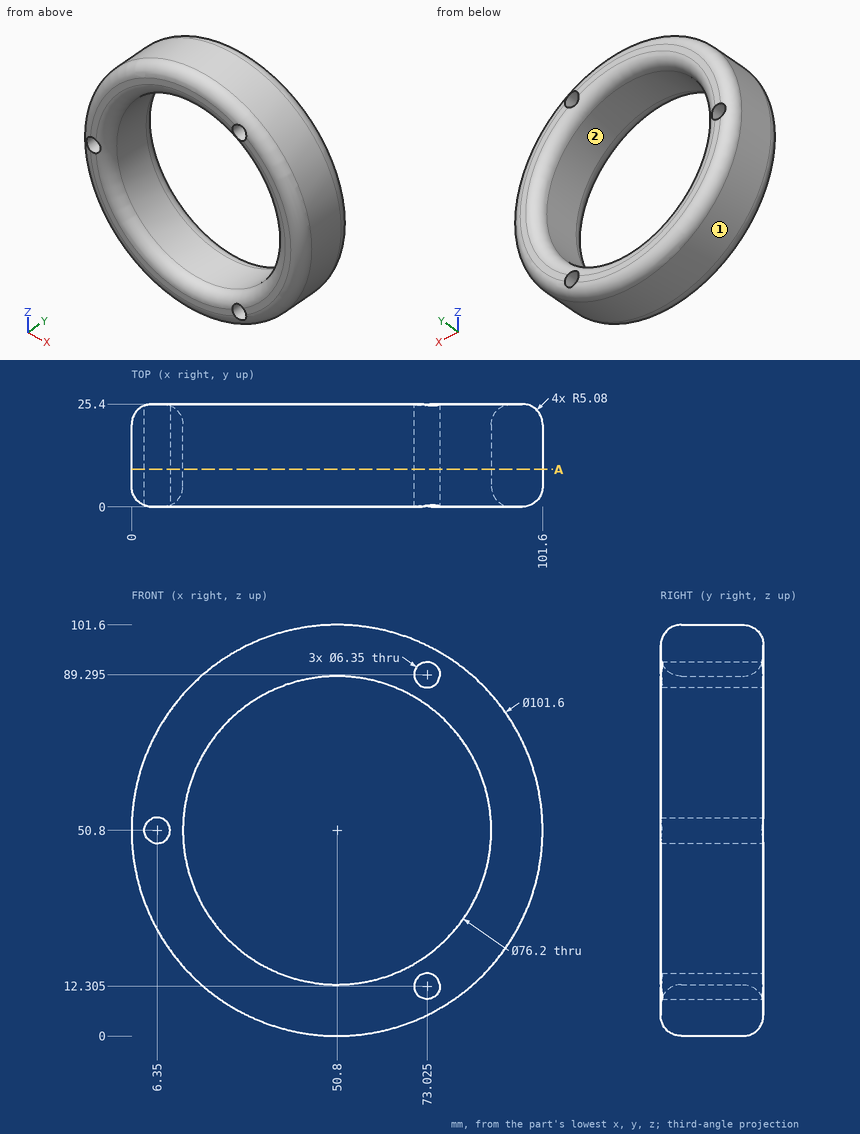
Source: three-view drawing plus pictorial views. Frame: mm from the lowest corner of the part. Give positions to 0.01 mm unless a question says otherwise; leave off trailing zeros. Write each question's results on one line, items separated by ' | '. Start each with the question number.
Item 1: Cut plane A-A on y = 9.25. Give the number of separate pieces and of enclosed holes in the cut face, then the cut area to 3 significant figures.
Item 2: Line query: line 1 (Z direction, x = 82.5, y = 17.25) (1 decimal); line 2 (X direction, y = 8.25, z = 21); line 3 (X direction, y = 15, z = 69.5) (1 decimal). Output: solid intervals per line, ascending.
Item 3: Contact query for flat-ended pins moving along their axis: P1, Ø1, axis at x = 13.5, y = 5.5, coming from the -Z side; P2, Ø2, axis at x = 45.5, y = 15, coming from the -Z side; P3, Ø4, axis at x = 54.5, y = 12, coming from the -Z side. Output: stop coordinate, or through.
Item 4: Mould query, pull axis X, two halves, no side actions, for the marked faces 1 and 2. Classes: pulls with the +X half, pulls with the -X half, needs draft (parallel to the pull), parting line crosses it, or undercut.
Established:
1) separate pieces: 1 | enclosed holes: 4 | area: 3,450 mm^2
2) line 1: 11.1 to 29.7, 71.9 to 90.5 | line 2: 9.66 to 27.06, 74.54 to 91.94 | line 3: 3.6 to 17.6, 84 to 98
3) P1: z = 15.78 | P2: z = 0.18 | P3: z = 0.03
4) face 1: parting line crosses it | face 2: undercut
